The model under review builds one solid part; all positions refer to its coordinate system, in mm. A direction names the side the tool comes from. Give positions to 0.01 mm unless a question says otherwise; leave off trailing zeros. Write each loop counter-clockwise with the first axis right and the second up, starting at its lowest first coordinate (ties: lowest second). Pieces come first, ordered by that corner, then holes.
from build123d import *

# Parameters (mm, degrees)
SKETCH1_W           = 80
SKETCH1_H           = 105
SKETCH1_W_2         = 60
SKETCH1_H_2         = 71.314940153
SKETCH1_R           = 2
BOSS_EXTRUDE2_DEPTH = 8
SKETCH2_W           = 72
SKETCH2_H           = 97
CUT_EXTRUDE1_DEPTH  = 6
SKETCH3_W           = 76
SKETCH3_H           = 101
BOSS_EXTRUDE3_DEPTH = 2
SKETCH4_W           = 72
SKETCH4_H           = 97
CUT_EXTRUDE2_DEPTH  = 2
SKETCH5_R           = 2.5
CUT_EXTRUDE3_DEPTH  = 5
FILLET1_R           = 2
SKETCH6_W           = 2
SKETCH6_H           = 18
CUT_EXTRUDE4_DEPTH  = 2


with BuildPart() as part:
    # Sketch1 → Boss-Extrude2 (new body)
    # profile 1 of 2: a face of its own
    with BuildSketch(Plane.XY):
        with Locations((35, -13.965517241)):
            Rectangle(SKETCH1_W, SKETCH1_H)
        with Locations((37, -26.808047164)):
            Rectangle(SKETCH1_W_2, SKETCH1_H_2, mode=Mode.SUBTRACT)
    # profile 2 of 2: a face of its own
    with BuildSketch(Plane.XY):
        with Locations((37, -26.808047164)):
            Rectangle(SKETCH1_W_2, SKETCH1_H_2)
        with Locations((14, -8.150577088)):
            Circle(SKETCH1_R, mode=Mode.SUBTRACT)
        with Locations((18.5, -57.465517241)):
            Circle(SKETCH1_R, mode=Mode.SUBTRACT)
        with Locations((46, -57.465517241)):
            Circle(SKETCH1_R, mode=Mode.SUBTRACT)
        with Locations((63, -8.950577088)):
            Circle(SKETCH1_R, mode=Mode.SUBTRACT)
    extrude(amount=BOSS_EXTRUDE2_DEPTH)

    # Sketch2 → Cut-Extrude1 (cut)
    with BuildSketch(Plane.XY.offset(8)):
        with Locations((35, -13.965517241)):
            Rectangle(SKETCH2_W, SKETCH2_H)
    extrude(amount=-CUT_EXTRUDE1_DEPTH, mode=Mode.SUBTRACT)

    # Sketch3 → Boss-Extrude3 (add)
    with BuildSketch(Plane.XY.offset(8)):
        with Locations((35, -13.965517241)):
            Rectangle(SKETCH3_W, SKETCH3_H)
    extrude(amount=BOSS_EXTRUDE3_DEPTH)

    # Sketch4 → Cut-Extrude2 (cut)
    with BuildSketch(Plane.XY.offset(10)):
        with Locations((35, -13.965517241)):
            Rectangle(SKETCH4_W, SKETCH4_H)
    extrude(amount=-CUT_EXTRUDE2_DEPTH, mode=Mode.SUBTRACT)

    # Sketch5 → Cut-Extrude3 (cut)
    with BuildSketch(Plane(origin=(0, -66.465517241, 0), x_dir=(-1, 0, 0), z_dir=(0, -1, 0))):
        with Locations((-35, -8)):
            Circle(SKETCH5_R)
    extrude(amount=-CUT_EXTRUDE3_DEPTH, mode=Mode.SUBTRACT)

    # Fillet1
    fillet1_edges = [part.edges().sort_by_distance(p)[0] for p in [
        (35, -66.465517241, 0),
        (-5, -13.965517241, 0),
        (35, 38.534482759, 0),
        (75, -13.965517241, 0),
    ]]
    fillet(fillet1_edges, radius=FILLET1_R)

    # Sketch6 → Cut-Extrude4 (cut)
    with BuildSketch(Plane.XY.offset(10)):
        with Locations((-2, 22.534482759)):
            Rectangle(SKETCH6_W, SKETCH6_H)
    extrude(amount=-CUT_EXTRUDE4_DEPTH, mode=Mode.SUBTRACT)


solid = part.part
1) Consider section D-D, the plane x = 51. Give the boundary of the cut face in (y, z), then the cut area to 3 significant figures.
2) The part is to be moulded in two halves that separate along X. For faces 1 (the flat face through (35, 37, 8)), 2 (the flat face through (34, 34.534, 6)), 3 (the cylindrical face through (62.566, -10.903, 0.986)), 4 (the cylindrical face through (-4.43, -13.23, 0.6)), say which applies: +X half, -X half, draft (parallel to the pull), parting line (faces both ways), or undercut.
3) To check wall thickness, follow probe 1 along X at (y, z) = (-51, 3.75); probe 2 along Y at (x, z) = (45, 3.75); probe 3 along X at (y, z) = (-56.5, 0.75). State the ranges of each line that lie inside material, in increasing order.
4) Consider section A-A, the plane x = 18.5. Give the boundary of the cut face in (y, z).
5) Tool access review of faces 5 (the flat face through (-2, 13.534, 9)), 6 (the flat face through (-3, -26, 9)), 7 (the flat face through (34, -13, 2)): name each direction out of +Z, -Z, +X, -X, +Y, -Y from which nothing blocks a thin tool from reaching the whole face with its end or side.
6) Insertion check: pin 1 (1 mm diameter, centred on x = 20.5, z = 9, fed in from +Y); pin 2 (4.5 mm diameter, centred on x = 46, y = -57.47, fed in from +Z); pin 3 (0.6 mm diameter, centred on y = 33.5, z = 9, fed in from -X). Each pin has a flat end and moves straight along its axis. Give the tip position at first contact, or say it passes through.
7) Consider section C-C, the plane y = 17. Give the boundary of the cut face in (x, z).
8) Consider section B-B, the plane z = 4. Give the boundary of the cut face in (x, y), then the cut area to 3 significant figures.
Answer block:
1. outline: (-66.47, 2) arc R2 ccw to (-64.47, 0) - (36.53, 0) arc R2 ccw to (38.53, 2) - (38.53, 8) - (36.53, 8) - (36.53, 10) - (34.53, 10) - (34.53, 2) - (-62.47, 2) - (-62.47, 10) - (-64.47, 10) - (-64.47, 8) - (-66.47, 8) - close
1. area: 264 mm2
2. face 1: draft
2. face 2: undercut
2. face 3: undercut
2. face 4: -X half
3. probe 1: x = -5 to -1, 71 to 75
3. probe 2: y = -66.47 to -62.47, 34.53 to 38.53
3. probe 3: x = -4.56 to 16.75, 20.25 to 44.25, 47.75 to 74.56
4. outline: (-66.47, 2) arc R2 ccw to (-64.47, 0) - (-59.47, 0) - (-59.47, 2) - (-62.47, 2) - (-62.47, 10) - (-64.47, 10) - (-64.47, 8) - (-66.47, 8) - close; (-55.47, 0) - (36.53, 0) arc R2 ccw to (38.53, 2) - (38.53, 8) - (36.53, 8) - (36.53, 10) - (34.53, 10) - (34.53, 2) - (-55.47, 2) - close
5. face 5: +Z, -X
5. face 6: +Z, -X, +Y, -Y
5. face 7: +Z
6. pin 1: stops at y = 36.53
6. pin 2: stops at z = 2
6. pin 3: stops at x = -3
7. outline: (-5, 2) arc R2 ccw to (-3, 0) - (73, 0) arc R2 ccw to (75, 2) - (75, 8) - (73, 8) - (73, 10) - (71, 10) - (71, 2) - (-1, 2) - (-1, 8) - (-5, 8) - close
8. outline: (-5, -66.47) - (75, -66.47) - (75, 38.53) - (-5, 38.53) - close; hole (-1, -62.47) - (71, -62.47) - (71, 34.53) - (-1, 34.53) - close
8. area: 1,420 mm2
